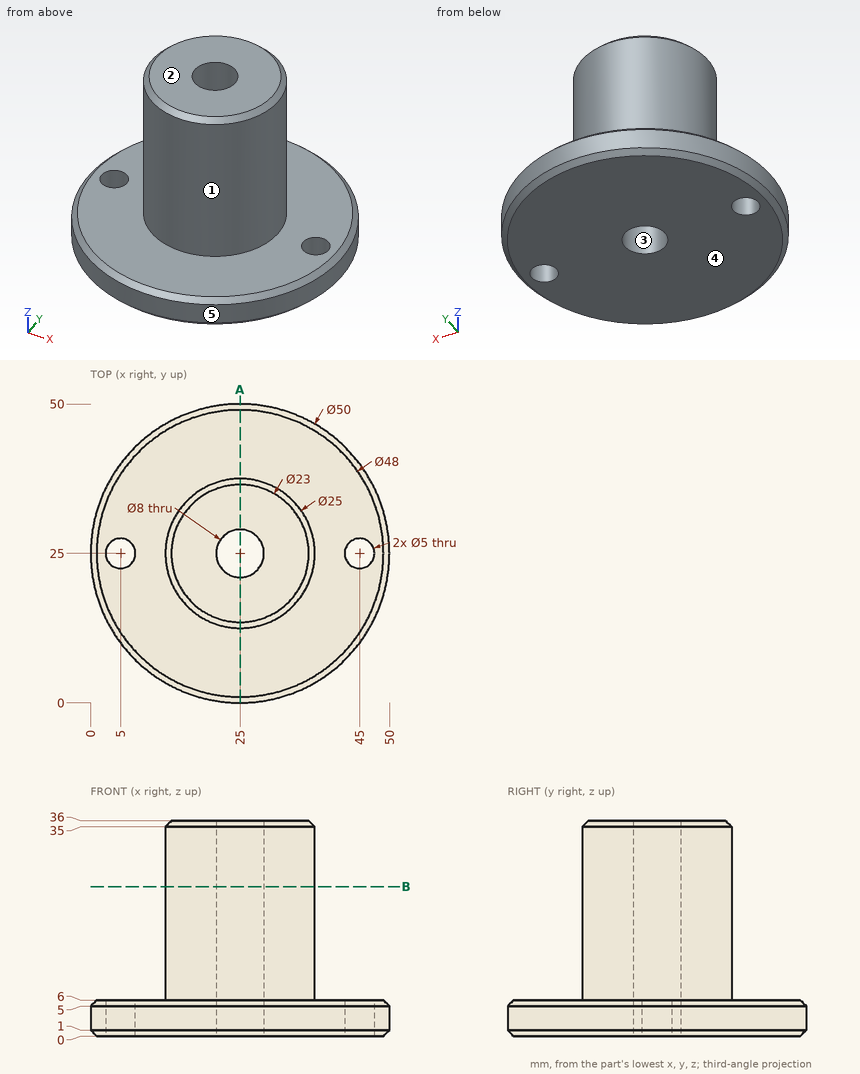
Geometry check sheet. Reference: drawing and pictorial views, mm from the part's lowest x, y, z. A direction names the side the tool comes from. Round coordinates to 2 decimals unless told otherwise and drop trailing zeros. Order: outer loops, then holes, each group sorted by start corner. A loop starts at its lowest first (then second) coordinate and runs counter-clockwise, first axis right, second up. Notation, with made-up numbers: M 20.25,68 L 45.25,68 A30 cw 45.25,91 Z; hole C -9.5,-24 d8. An arc over 180 degrees is marked long. One line per item, written item: value. Start each with the question number.
1. Release check for a two-part mould opening along Y. For the marked faces 3, 4 and 5 record: released by +Y, released by -Y, zero draft, split by the parting line, or undercut.
2. Scan lines: line 1 along Y through (x, z) = (25, 18); line 2 along Z through (x, y) = (38, 7); line 3 along Y through (x, z) = (5, 3.15). Record each from-to range of solid material in increasing order.
3. Section check A-A on x = 25. Enter the section's corners in (y, z).
4. Section check B-B on z = 25. Enter the section's corners in (x, y), and give its area (3 significant figures).
5. Gauge pin test, flat ends, axial feed: P1, Ø6, axis at y = 27, z = 7, coming from the +X side; P2, Ø1.5, axis at x = 33.5, z = 22, coming from the -Y side; P3, Ø8, axis at y = 39.5, z = 13.5, coming from the -X side; P4, Ø6, axis at y = 28, z = 19, coming from the -X side. Record the tip position at first contact, or that the pin passes through.
6. Access from +Z, -Z, +X, -X, +Y, -Y to the whole of each face (thin tool, end or side, straight path). Record for the marked faces 1 and 2.
Results found:
1. face 3: undercut
1. face 4: zero draft
1. face 5: split by the parting line
2. line 1: 12.5 to 21, 29 to 37.5
2. line 2: 0 to 6
2. line 3: 10 to 22.5, 27.5 to 40
3. outline: M 0,1 L 1,0 L 21,0 L 21,36 L 13.5,36 L 12.5,35 L 12.5,6 L 1,6 L 0,5 Z; M 29,0 L 49,0 L 50,1 L 50,5 L 49,6 L 37.5,6 L 37.5,35 L 36.5,36 L 29,36 Z
4. outline: C 25,25 d25; hole C 25,25 d8
4. area: 441 mm^2
5. P1: x = 50
5. P2: y = 15.19
5. P3: x = 18.22
5. P4: x = 12.5
6. face 1: +Z
6. face 2: +Z, +X, -X, +Y, -Y
